Check sheet for the drawn part. Datum: minimum x, y, z corner. Units: mm. Give positions to 0.01 mm unless a question says otherwise; leave off trailing zeros. Order: outer loops, then holes, each group sorted by start corner. A loop starts at its lowest first (then second) coordinate and runs counter-clockwise, first axis right, second up. Notation, with made-up numbers: (-26.75, 71) -> (14.25, 71) arc R25 cw to (14.25, 101) -> close; hole circle Ø8 at (29, 47). An arc over 180 degrees is marked (long way). One line per question, with ' | ' between items. Start each with the question number.
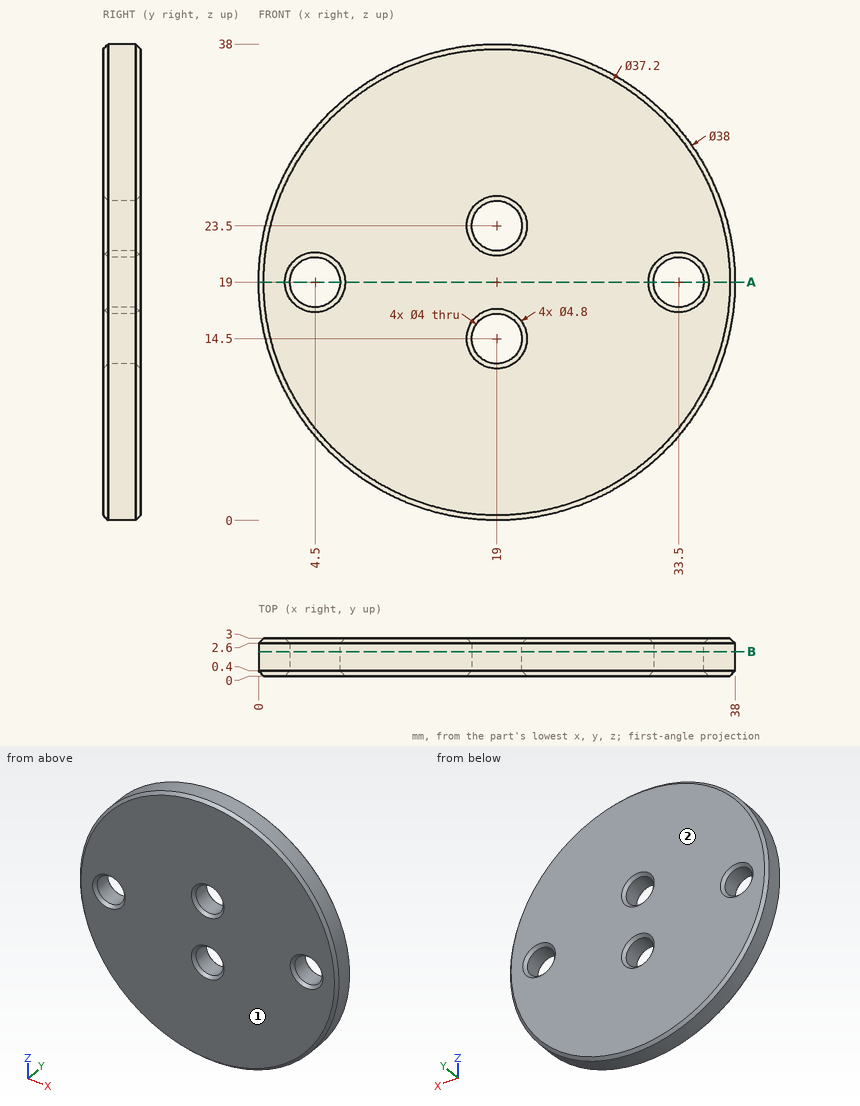
1. Cross-section at B-B on y = 1.95. Record the boundary of the cut face in (x, z), and give its area (3 significant figures).
2. Cross-section at A-A on z = 19. Record the boundary of the cut face in (x, y).
3. Scan lines: probe 1 along X at (y, z) = (2.1, 19); probe 2 along Z at (x, y) = (19, 0.85); probe 3 along Z at (x, y) = (28, 2.8). Record each from-to range of solid material in increasing order.
4. Go/stop test with flat-tipped pins: pin 1 (3.5 mm diameter, centred on x = 4.5, z = 19, fed in from -Y); pin 2 (8 mm diameter, centred on x = 8, z = 4, fed in from -Y). Record where each tip stops, or that it passes through.
5. Mould release check, pull along Y, two halves, no side actions. Record for the marked faces 1 and 2: +Y half, -Y half, draft (parallel to the pull), parting line (faces both ways), or undercut.
Response values:
1) outline: circle Ø38 at (19, 19); hole circle Ø4 at (4.5, 19); hole circle Ø4 at (19, 14.5); hole circle Ø4 at (19, 23.5); hole circle Ø4 at (33.5, 19) | area: 1,080 mm²
2) outline: (0, 0.4) -> (0.4, 0) -> (2.1, 0) -> (2.5, 0.4) -> (2.5, 2.6) -> (2.1, 3) -> (0.4, 3) -> (0, 2.6) -> close; (6.5, 0.4) -> (6.9, 0) -> (31.1, 0) -> (31.5, 0.4) -> (31.5, 2.6) -> (31.1, 3) -> (6.9, 3) -> (6.5, 2.6) -> close; (35.5, 0.4) -> (35.9, 0) -> (37.6, 0) -> (38, 0.4) -> (38, 2.6) -> (37.6, 3) -> (35.9, 3) -> (35.5, 2.6) -> close
3) probe 1: x = 0 to 2.5, 6.5 to 31.5, 35.5 to 38 | probe 2: z = 0 to 12.5, 16.5 to 21.5, 25.5 to 38 | probe 3: z = 2.49 to 35.51
4) pin 1: passes through | pin 2: stops at y = 0
5) face 1: -Y half | face 2: +Y half
